The listing builds one solid part. Answer for the finished solid, in the listing's coordinates (mm). A direction names the side the tool comes from. Round coordinates to 2 decimals unless told otherwise and drop trailing zeros. Write each loop counter-clockwise with the first axis right and the second up, starting at its lowest first coordinate (ties: lowest second). Pieces come first, ordered by that corner, then holes.
(1) For faces 4 (the face through (64, 13, -25.5)), 5 (the face through (73, 14, 44)), 6 (the face through (52.5, 6, 26)), determine the directions among +Z, -Z, +X, -X, +Y, -Y from which every point of the face is accessible in a straight line to the end or side of a thin tool.
(2) The mould has two halves that part along Y. Classify faces 1 (the face through (-21, 3, -37)), 2 (the face through (-31, 6, 35)), 3 (the face through (-31, 20, 36)): +Y half, -Y half, draft (parallel to the pull), parting line (faces both ways), or undercut.
(3) Each of these flat-tipped pins is pushed along its axis until it touches: pin 1 Ø6 at (x, z) = (-32.5, 4.5) entering from +Y; pin 2 Ø4.5 at (x, z) = (59, 36.5) entering from +Y; pin 3 Ø1 at (x, z) = (65.5, 11.5) entering from +Y. Where does it stop, or does it pass through?
(4) A cutting plane is placed at C-C, the plane z = 35.35. Give the number of separate pieces and of enclosed holes in the cut face, and give its area (3 significant figures).
(5) A cutting plane is placed at B-B, the plane z = -19. Give the vertices of the cut face in (x, y).
(6) Find the intervals of material crossed by probe 1 along Z at (x, y) = (32.5, 3.5); probe 2 along Z at (x, y) = (-55.5, 14.75); probe 3 along X at (y, z) = (6.75, 36), in increasing order.
from build123d import *

# Parameters (mm, degrees)
CROQUIS1_W              = 150
CROQUIS1_H              = 90
SALIENTE_EXTRUIR1_DEPTH = 3
SALIENTE_EXTRUIR2_DEPTH = 25
CROQUIS3_W              = 38
CROQUIS3_H              = 2
CROQUIS3_W_2            = 23
SALIENTE_EXTRUIR3_DEPTH = 14
SALIENTE_EXTRUIR4_START = 6
CROQUIS4_W              = 38
CROQUIS4_H              = 15.3
CROQUIS4_R              = 1.5
CROQUIS4_W_2            = 23
SALIENTE_EXTRUIR4_DEPTH = 3
CORTAR_EXTRUIR1_REACH   = 110.14
CROQUIS5_W              = 20
CROQUIS5_H              = 6
CROQUIS5_W_2            = 10
REDONDEO1_R             = 15
REDONDEO2_R             = 5
SALIENTE_EXTRUIR5_START = 25
SALIENTE_EXTRUIR5_DEPTH = 25
CROQUIS7_R              = 3.6
CORTAR_EXTRUIR2_DEPTH   = 2
CROQUIS8_W              = 9.129710912
CROQUIS8_H              = 9.129710912
CROQUIS8_W_2            = 5.7
CROQUIS8_H_2            = 5.7
SALIENTE_EXTRUIR6_DEPTH = 2
CROQUIS9_W              = 15
CROQUIS9_H              = 2
SALIENTE_EXTRUIR7_DEPTH = 20


with BuildPart() as part:
    # Croquis1 → Saliente-Extruir1 (new body)
    with BuildSketch(Plane(origin=(0, 0, 0), x_dir=(1, 0, 0), z_dir=(0, 1, 0))):
        Rectangle(CROQUIS1_W, CROQUIS1_H)
    extrude(amount=SALIENTE_EXTRUIR1_DEPTH)

    # Croquis2 → Saliente-Extruir2 (add)
    with BuildSketch(Plane(origin=(0, 3, 0), x_dir=(1, 0, 0), z_dir=(0, 1, 0))):
        Polygon((-75, -45), (-75, 45), (75, 45), (75, -45), (69, -45), (69, -27.7), (46, -27.7), (46, -45), (-31, -45), (-31, -27.7), (-69, -27.7), (-69, -45), align=None)
        Polygon((-72, 42), (72, 42), (72, -24.7), (43, -24.7), (43, -42), (-28, -42), (-28, -24.7), (-72, -24.7), align=None, mode=Mode.SUBTRACT)
    extrude(amount=SALIENTE_EXTRUIR2_DEPTH)

    # Croquis3 → Saliente-Extruir3 (add)
    with BuildSketch(Plane(origin=(0, 3, 0), x_dir=(1, 0, 0), z_dir=(0, 1, 0))):
        with Locations((-50, -44)):
            Rectangle(CROQUIS3_W, CROQUIS3_H)
        with Locations((57.5, -44)):
            Rectangle(CROQUIS3_W_2, CROQUIS3_H)
    extrude(amount=SALIENTE_EXTRUIR3_DEPTH)

    # Croquis4 → Saliente-Extruir4 (add)
    # profile 1 of 2: a face of its own
    with BuildSketch(Plane(origin=(0, 3, 0), x_dir=(1, 0, 0), z_dir=(0, 1, 0)).offset(SALIENTE_EXTRUIR4_START)):
        with Locations((-50, -35.35)):
            Rectangle(CROQUIS4_W, CROQUIS4_H)
        with Locations(Location((-50, -35.35, 0), (0, 0, 270))):
            Circle(CROQUIS4_R, mode=Mode.SUBTRACT)
        with Locations(Location((-40, -35.35, 0), (0, 0, 270))):
            Circle(CROQUIS4_R, mode=Mode.SUBTRACT)
        with Locations(Location((-60, -35.35, 0), (0, 0, 270))):
            Circle(CROQUIS4_R, mode=Mode.SUBTRACT)
    # profile 2 of 2: a face of its own
    with BuildSketch(Plane(origin=(0, 3, 0), x_dir=(1, 0, 0), z_dir=(0, 1, 0)).offset(SALIENTE_EXTRUIR4_START)):
        with Locations((57.5, -35.35)):
            Rectangle(CROQUIS4_W_2, CROQUIS4_H)
        with Locations(Location((62.5, -35.35, 0), (0, 0, 270))):
            Circle(CROQUIS4_R, mode=Mode.SUBTRACT)
        with Locations(Location((52.5, -35.35, 0), (0, 0, 270))):
            Circle(CROQUIS4_R, mode=Mode.SUBTRACT)
    extrude(amount=SALIENTE_EXTRUIR4_DEPTH)

    # Croquis5 → Cortar-Extruir1 (cut, up to next)
    with BuildSketch(Plane.XY.offset(27.7), mode=Mode.PRIVATE) as cortar_extruir1_sk1:
        with Locations((-50, 6)):
            Rectangle(CROQUIS5_W, CROQUIS5_H)
    cortar_extruir1_tool1 = extrude(cortar_extruir1_sk1.sketch, amount=-CORTAR_EXTRUIR1_REACH, mode=Mode.PRIVATE) & part.part
    # Croquis5 → Cortar-Extruir1 (cut, up to next)
    with BuildSketch(Plane.XY.offset(27.7), mode=Mode.PRIVATE) as cortar_extruir1_sk2:
        with Locations((57.5, 6)):
            Rectangle(CROQUIS5_W_2, CROQUIS5_H)
    cortar_extruir1_tool2 = extrude(cortar_extruir1_sk2.sketch, amount=-CORTAR_EXTRUIR1_REACH, mode=Mode.PRIVATE) & part.part
    add(cortar_extruir1_tool1.solids().sort_by_distance((-50, 6, 27.7))[0], mode=Mode.SUBTRACT)
    add(cortar_extruir1_tool2.solids().sort_by_distance((57.5, 6, 27.7))[0], mode=Mode.SUBTRACT)

    # Redondeo1
    redondeo1_edges = [part.edges().sort_by_distance(p)[0] for p in [
        (72, 15.5, -42),
        (-72, 15.5, -42),
        (-75, 14, -45),
        (75, 14, -45),
    ]]
    fillet(redondeo1_edges, radius=REDONDEO1_R)

    # Redondeo2
    redondeo2_edges = [part.edges().sort_by_distance(p)[0] for p in [
        (75, 14, 45),
        (-75, 14, 45),
    ]]
    fillet(redondeo2_edges, radius=REDONDEO2_R)

    # Croquis6 → Saliente-Extruir5 (add)
    with BuildSketch(Plane(origin=(0, 3, 0), x_dir=(1, 0, 0), z_dir=(0, 1, 0)).offset(SALIENTE_EXTRUIR5_START)):
        with BuildLine():
            Line((-64.071067812, 39.071067812), (-65.90445517, 39.071067812))
            ThreePointArc((-65.90445517, 39.071067812), (-67.606601718, 37.606601718), (-69.071067812, 35.90445517))
            Line((-69.071067812, 35.90445517), (-69.071067812, 34.071067812))
            ThreePointArc((-69.071067812, 34.071067812), (-60.535533906, 30.535533906), (-64.071067812, 39.071067812))
        make_face()
        with BuildLine():
            Line((-67, -24.7), (-72, -24.7))
            Line((-72, -24.7), (-72, -19.7))
            ThreePointArc((-72, -19.7), (-63.464466094, -16.164466094), (-67, -24.7))
        make_face()
        with BuildLine():
            Line((72, -24.7), (72, -19.7))
            ThreePointArc((72, -19.7), (63.464466094, -16.164466094), (67, -24.7))
            Line((67, -24.7), (72, -24.7))
        make_face()
        with BuildLine():
            Line((69.071067812, 34.071067812), (69.071067812, 35.90445517))
            ThreePointArc((69.071067812, 35.90445517), (67.606601718, 37.606601718), (65.90445517, 39.071067812))
            Line((65.90445517, 39.071067812), (64.071067812, 39.071067812))
            ThreePointArc((64.071067812, 39.071067812), (60.535533906, 30.535533906), (69.071067812, 34.071067812))
        make_face()
    extrude(amount=-SALIENTE_EXTRUIR5_DEPTH)

    # Croquis7 → Cortar-Extruir2 (cut)
    with BuildSketch(Plane(origin=(0, 28, 0), x_dir=(1, 0, 0), z_dir=(0, 1, 0))):
        with Locations(Location((-64.071067812, 34.071067812, 0), (0, 0, 270))):
            Circle(CROQUIS7_R)
        with Locations(Location((64.071067812, 34.071067812, 0), (0, 0, 270))):
            Circle(CROQUIS7_R)
        with Locations(Location((67, -19.7, 0), (0, 0, 270))):
            Circle(CROQUIS7_R)
        with Locations(Location((-67, -19.7, 0), (0, 0, 270))):
            Circle(CROQUIS7_R)
    extrude(amount=-CORTAR_EXTRUIR2_DEPTH, mode=Mode.SUBTRACT)

    # Croquis8 → Saliente-Extruir6 (add)
    # profile 1 of 8: a face of its own
    with BuildSketch(Plane(origin=(0, 3, 0), x_dir=(1, 0, 0), z_dir=(0, 1, 0))):
        with Locations((-34.25, 25)):
            Rectangle(CROQUIS8_W, CROQUIS8_H)
        with Locations((-34.25, 25)):
            Rectangle(CROQUIS8_W_2, CROQUIS8_H_2, mode=Mode.SUBTRACT)
    # profile 2 of 8: a face of its own
    with BuildSketch(Plane(origin=(0, 3, 0), x_dir=(1, 0, 0), z_dir=(0, 1, 0))):
        with Locations((-55.75, 25)):
            Rectangle(CROQUIS8_W, CROQUIS8_H)
        with Locations((-55.75, 25)):
            Rectangle(CROQUIS8_W_2, CROQUIS8_H_2, mode=Mode.SUBTRACT)
    # profile 3 of 8: a face of its own
    with BuildSketch(Plane(origin=(0, 3, 0), x_dir=(1, 0, 0), z_dir=(0, 1, 0))):
        with Locations((-34.25, -13)):
            Rectangle(CROQUIS8_W, CROQUIS8_H)
        with Locations((-34.25, -13)):
            Rectangle(CROQUIS8_W_2, CROQUIS8_H_2, mode=Mode.SUBTRACT)
    # profile 4 of 8: a face of its own
    with BuildSketch(Plane(origin=(0, 3, 0), x_dir=(1, 0, 0), z_dir=(0, 1, 0))):
        with Locations((-55.75, -13)):
            Rectangle(CROQUIS8_W, CROQUIS8_H)
        with Locations((-55.75, -13)):
            Rectangle(CROQUIS8_W_2, CROQUIS8_H_2, mode=Mode.SUBTRACT)
    # profile 5 of 8: a face of its own
    with BuildSketch(Plane(origin=(0, 3, 0), x_dir=(1, 0, 0), z_dir=(0, 1, 0))):
        with Locations((36, 37)):
            Rectangle(CROQUIS8_W, CROQUIS8_H)
        with Locations((36, 37)):
            Rectangle(CROQUIS8_W_2, CROQUIS8_H_2, mode=Mode.SUBTRACT)
    # profile 6 of 8: a face of its own
    with BuildSketch(Plane(origin=(0, 3, 0), x_dir=(1, 0, 0), z_dir=(0, 1, 0))):
        with Locations((-21, 37)):
            Rectangle(CROQUIS8_W, CROQUIS8_H)
        with Locations((-21, 37)):
            Rectangle(CROQUIS8_W_2, CROQUIS8_H_2, mode=Mode.SUBTRACT)
    # profile 7 of 8: a face of its own
    with BuildSketch(Plane(origin=(0, 3, 0), x_dir=(1, 0, 0), z_dir=(0, 1, 0))):
        with Locations((-21, -34)):
            Rectangle(CROQUIS8_W, CROQUIS8_H)
        with Locations((-21, -34)):
            Rectangle(CROQUIS8_W_2, CROQUIS8_H_2, mode=Mode.SUBTRACT)
    # profile 8 of 8: a face of its own
    with BuildSketch(Plane(origin=(0, 3, 0), x_dir=(1, 0, 0), z_dir=(0, 1, 0))):
        with Locations((36, -34)):
            Rectangle(CROQUIS8_W, CROQUIS8_H)
        with Locations((36, -34)):
            Rectangle(CROQUIS8_W_2, CROQUIS8_H_2, mode=Mode.SUBTRACT)
    extrude(amount=SALIENTE_EXTRUIR6_DEPTH)

    # Croquis9 → Saliente-Extruir7 (add)
    with BuildSketch(Plane(origin=(0, 3, 0), x_dir=(1, 0, 0), z_dir=(0, 1, 0))):
        with Locations((64.5, -11.7)):
            Rectangle(CROQUIS9_W, CROQUIS9_H)
        with Locations((64.5, 24.5)):
            Rectangle(CROQUIS9_W, CROQUIS9_H)
    extrude(amount=SALIENTE_EXTRUIR7_DEPTH)


solid = part.part
Solutions:
1. face 4: +Y
1. face 5: +Z, +X, +Y, -Y
1. face 6: none
2. face 1: +Y half
2. face 2: undercut
2. face 3: draft
3. pin 1: stops at y = 3
3. pin 2: stops at y = 12
3. pin 3: stops at y = 23
4. separate pieces: 4
4. enclosed holes: 0
4. area: 1,050 mm2
5. outline: (-75, 0) - (75, 0) - (75, 28) - (72, 28) - (72, 3) - (-72, 3) - (-72, 28) - (-75, 28) - close
6. probe 1: z = -45 to -42, -41.56 to -32.44, 29.44 to 38.56, 42 to 45
6. probe 2: z = -45 to -42, 24.7 to 27.7, 43 to 45
6. probe 3: x = -75 to -69, -31 to -28, 43 to 46, 69 to 75
